Check sheet for the modelled part. Datum: model origin and axes. Units: mm. A direction names the side the tool comes from. Coordinates: 2 decimals unless noted, no trailing zeros. Loops run counter-clockwise (first coordinate to the right, second up) from the corner with the lowest first, then second, coordinate; pieces in that order, holes last. Notation, with made-up numbers: M -18.5,69.5 L 38.5,69.5 A20 ccw 38.5,87.5 Z; hole C 12.5,66.25 d7. An arc over 180 degrees is marked long. Return JSON: item names as keys, results as strings.
from build123d import *

# Parameters (mm, degrees)
SKETCH1_R           = 2
BOSS_EXTRUDE1_DEPTH = 12
SKETCH2_W           = 20.5
SKETCH2_H           = 20.5
CUT_EXTRUDE1_DEPTH  = 5
SKETCH4_R           = 3.45
CUT_EXTRUDE7_DEPTH  = 8


with BuildPart() as part:
    # Sketch1 → Boss-Extrude1 (new body)
    with BuildSketch(Plane.XY):
        Polygon((0, 0), (69.7, 0), (90.3, 0), (160, 0), (160, 70), (164, 70), (164, 90), (160, 90), (160, 160), (90, 160), (90, 164), (70, 164), (70, 160), (0, 160), (0, 90.3), (0, 69.7), align=None)
        with Locations((151.5, 133.3)):
            Circle(SKETCH1_R, mode=Mode.SUBTRACT)
    extrude(amount=BOSS_EXTRUDE1_DEPTH)

    # Sketch2 → Cut-Extrude1 (cut)
    with BuildSketch(Plane.XY.offset(12)):
        with Locations((15, 15)):
            Rectangle(SKETCH2_W, SKETCH2_H)
    extrude(amount=-CUT_EXTRUDE1_DEPTH, mode=Mode.SUBTRACT)

    # Sketch4 → Cut-Extrude7 (cut)
    with BuildSketch(Plane(origin=(0, 0, 0), x_dir=(-1, 0, 0), z_dir=(0, 0, -1))):
        with Locations((-151.5, 133.3)):
            Circle(SKETCH4_R)
    extrude(amount=-CUT_EXTRUDE7_DEPTH, mode=Mode.SUBTRACT)


solid = part.part
1) Section check D-D on z = 3. Record the cut outline in (x, y), then the cut area to 3 significant figures.
Answers:
{"outline": "M 0,0 L 160,0 L 160,70 L 164,70 L 164,90 L 160,90 L 160,160 L 90,160 L 90,164 L 70,164 L 70,160 L 0,160 Z; hole C 151.5,133.3 d6.9", "area": "25,700 mm²"}
2) Go/stop test with flat-tipped pins: pin 1 Ø3.5 at (x, y) = (151.5, 133.3) entering from +Z (3 decimals); pin 2 Ø3 at (x, z) = (162.5, 7.5) entering from +Y; pin 3 Ø1.5 at (x, z) = (13.5, 9.5) entering from +Y; pin 4 Ø3 at (y, z) = (162.5, 7) entering from +X. Record where each tip stops, or that it passes through.
Answers:
{"pin 1": "through", "pin 2": "y = 90", "pin 3": "y = 160", "pin 4": "x = 90"}
3) Section check A-A on x = 151.5. Record the cut outline in (y, z).
Answers:
{"outline": "M 0,0 L 129.85,0 L 129.85,8 L 131.3,8 L 131.3,12 L 0,12 Z; M 135.3,8 L 136.75,8 L 136.75,0 L 160,0 L 160,12 L 135.3,12 Z"}
4) Section check C-C on x = 21. Record the cut outline in (y, z), then the cut area to 3 significant figures.
Answers:
{"outline": "M 0,0 L 160,0 L 160,12 L 25.25,12 L 25.25,7 L 4.75,7 L 4.75,12 L 0,12 Z", "area": "1,820 mm²"}
5) Section check B-B on y = 133.3. Record the cut outline in (x, z), then the cut area to 3 significant figures.
Answers:
{"outline": "M 0,0 L 148.05,0 L 148.05,8 L 149.5,8 L 149.5,12 L 0,12 Z; M 153.5,8 L 154.95,8 L 154.95,0 L 160,0 L 160,12 L 153.5,12 Z", "area": "1,850 mm²"}
6) Scan lines: line 1 along X through (y, z) = (133.3, 3.5); line 2 along Y through (x, z) = (151.5, 3.5); line 3 along Y through (x, z) = (18.5, 9.5). Record each from-to range of solid material in increasing order. Write a range as [from, to].
Answers:
{"line 1": "[0, 148.05], [154.95, 160]", "line 2": "[0, 129.85], [136.75, 160]", "line 3": "[0, 4.75], [25.25, 160]"}
7) Set-up check for faces 1 (the face through (15, 15, 7)), 2 (the face through (70, 162, 6)), 3 (the face through (160, 35, 6)), 4 (the face through (160, 125, 6)), 5 (the face through (152, 131, 8)): record each of +Z, -Z, +X, -X, +Y, -Y from which the full face is reachable in a straight line by a thin tool's end or side.
Answers:
{"face 1": "+Z", "face 2": "+Z, -Z, -X, +Y", "face 3": "+Z, -Z, +X, -Y", "face 4": "+Z, -Z, +X, +Y", "face 5": "-Z"}
8) Draft check along Y on faces 6 (the face through (81, 83, 12)), 7 (the face through (15, 25.25, 10)), 8 (the face through (35, 160, 6)). Enter one of: +Y half, -Y half, draft (parallel to the pull), parting line (faces both ways), or undercut.
Answers:
{"face 6": "draft", "face 7": "undercut", "face 8": "+Y half"}
